```python
from build123d import *

# Parameters (mm, degrees)
SKETCH1_R                = 6.366
SKETCH1_R_2              = 3.175
BOSS_EXTRUDE1_DEPTH      = 10
BOSS_EXTRUDE2_START      = -2
SKETCH2_R                = 7.5
SKETCH2_R_2              = 3.175
BOSS_EXTRUDE2_DEPTH      = 2
BOSS_EXTRUDE3_DEPTH      = 5
BOSS_EXTRUDE3_DEPTH_BACK = 2
SKETCH3_R                = 7.5
SKETCH3_R_2              = 3.175


with BuildPart() as part:
    # Sketch1 → Boss-Extrude1 (new body)
    with BuildSketch(Plane(origin=(0, 0, 0), x_dir=(1, 0, 0), z_dir=(0, 1, 0))):
        with Locations(Location((0, 0, 0), (0, 0, 270))):
            Circle(SKETCH1_R)
        with Locations(Location((0, 0, 0), (0, 0, 270))):
            Circle(SKETCH1_R_2, mode=Mode.SUBTRACT)
    extrude(amount=BOSS_EXTRUDE1_DEPTH)

    # Sketch2 → Boss-Extrude2 (add)
    with BuildSketch(Plane(origin=(0, 10, 0), x_dir=(1, 0, 0), z_dir=(0, 1, 0)).offset(BOSS_EXTRUDE2_START)):
        with Locations(Location((0, 0, 0), (0, 0, 270))):
            Circle(SKETCH2_R)
        with Locations(Location((0, 0, 0), (0, 0, 270))):
            Circle(SKETCH2_R_2, mode=Mode.SUBTRACT)
    extrude(amount=BOSS_EXTRUDE2_DEPTH)

    # Sketch3 → Boss-Extrude3 (add, two sides: drawn at the far end of the back side and taken through both)
    with BuildSketch(Plane.XZ.offset(-BOSS_EXTRUDE3_DEPTH_BACK)):
        with Locations(Location((0, 0, 0), (0, 0, 90))):
            Circle(SKETCH3_R)
        with Locations(Location((0, 0, 0), (0, 0, 270))):
            Circle(SKETCH3_R_2, mode=Mode.SUBTRACT)
    extrude(amount=BOSS_EXTRUDE3_DEPTH + BOSS_EXTRUDE3_DEPTH_BACK)


solid = part.part
```
Verification items for the finished model (mm, model axes). A direction names the side the tool comes from. Give positions to 0.01 mm unless a question says otherwise; leave off trailing zeros. Loops run counter-clockwise (first coordinate to the right, second up) from the corner with the lowest first, then second, coordinate; pieces in that order, holes last. Notation, with made-up numbers: M 76.5,37.5 L 114.5,37.5 A35 cw 114.5,69.5 Z; hole C 51,23.25 d5. An arc over 180 degrees is marked long. Return JSON: item names as keys, results as strings.
1) Gauge pin test, flat end, axial feed: P1, Ø4, axis at x = 5.5, y = 7, coming from the +Z side. Record the tip position at first contact, or that the pin passes through.
Findings:
{"P1": "stops at z = 6.48"}
2) Section check B-B, the plane x = -1.5. Enter the section's corners in (y, z).
Findings:
{"outline": "M -5,-7.35 L 2,-7.35 L 2,-6.19 L 8,-6.19 L 8,-7.35 L 10,-7.35 L 10,-2.8 L -5,-2.8 Z; M -5,2.8 L 10,2.8 L 10,7.35 L 8,7.35 L 8,6.19 L 2,6.19 L 2,7.35 L -5,7.35 Z"}
3) Material ranges on L1, parallel to X at y = -2.7, z = 0 (3 decimals); L2, parallel to Z at x = 0, y = 4.25 (3 decimals), recorded low to high. Write a range as [from, to].
Findings:
{"L1": "x = [-7.5, -3.175], [3.175, 7.5]", "L2": "z = [-6.366, -3.175], [3.175, 6.366]"}
4) Section check A-A, the plane z = 0. Enter the section's corners in (x, y) (3 decimals), and give its area (3 significant figures).
Findings:
{"outline": "M -7.5,-5 L -3.175,-5 L -3.175,10 L -7.5,10 L -7.5,8 L -6.366,8 L -6.366,2 L -7.5,2 Z; M 3.175,-5 L 7.5,-5 L 7.5,2 L 6.366,2 L 6.366,8 L 7.5,8 L 7.5,10 L 3.175,10 Z", "area": "116 mm2"}
5) Tool access check on faces 4 (the cylindrical face through (-0.33, -1.451, -7.493)), 5 (the flat face through (-6, 8, -3)). Record the directions out of +Z, -Z, +X, -X, +Y, -Y that give a thin tool (end or side, any length) a straight path to the whole face; none if there is none.
Findings:
{"face 4": "+Y, -Y", "face 5": "none"}
6) Section check D-D, the plane z = 4.75. Enter the section's corners in (x, y), and give its area (3 significant figures).
Findings:
{"outline": "M -5.8,-5 L 5.8,-5 L 5.8,2 L 4.24,2 L 4.24,8 L 5.8,8 L 5.8,10 L -5.8,10 L -5.8,8 L -4.24,8 L -4.24,2 L -5.8,2 Z", "area": "155 mm2"}
7) Section check C-C, the plane y = 3. Enter the section's corners in (x, z) (3 decimals), and give its area (3 significant figures).
Findings:
{"outline": "C 0,0 d12.732; hole C 0,0 d6.35", "area": "95.6 mm2"}
8) Mould release check, pull along Y, two halves, no side actions. Record for faces 1 (the cylindrical face through (-3.874, 4.958, -5.052)), 2 (the cylindrical face through (0.33, 8.986, -7.493)), 3 (the flat face through (2, -5, 3)): released by +Y, released by -Y, zero draft, split by the parting line, or undercut.
Findings:
{"face 1": "undercut", "face 2": "zero draft", "face 3": "released by -Y"}
